Check sheet for the modelled part. Datum: model origin and axes. Units: mm. A direction names the side the tool comes from. Give positions to 0.01 mm unless a question says otherwise; leave off trailing zeros. Order: outer loops, then holes, each group sorted by start corner. A loop starts at its lowest first (then second) coordinate and runs counter-clockwise, first axis right, second up. Notation, with made-up numbers: (8.25, 25.25) -> (65.25, 25.25) arc R15 ccw to (65.25, 52.25) -> close; hole circle Ø9 at (73.25, 88.5). An arc over 180 degrees is marked (long way). One line per question, with ' | ' between items. Start each with the question number.
from build123d import *

# Parameters (mm, degrees)
SKETCH1_W                   = 50.8
SKETCH1_H                   = 50.8
STOCK_BLOCK_DEPTH           = 12.7
SKETCH2_R                   = 9.525
SLEEVE_NUT_HOLE_LARGE_DEPTH = 44.994090512
SKETCH11_W                  = 14.2875
SKETCH11_H                  = 50.8
CUT_EXTRUDE4_DEPTH          = 44.994090512
SKETCH3_W                   = 26.9875
SKETCH3_H                   = 12.7
CUT_EXTRUDE2_DEPTH          = 44.994090512
F_10_CLEARANCE_HOLE1_D      = 5.1054
SKETCH6_W                   = 3.175
SKETCH6_H                   = 37.090012852
CUT_EXTRUDE3_DEPTH          = 24.13
F_10_CLEARANCE_HOLE2_D      = 5.1054


with BuildPart() as part:
    # Sketch1 → Stock block (new, symmetric)
    with BuildSketch(Plane(origin=(0, 0, 0), x_dir=(1, 0, 0), z_dir=(0, 1, 0))):
        Rectangle(SKETCH1_W, SKETCH1_H)
    extrude(amount=STOCK_BLOCK_DEPTH, both=True)

    # Sketch2 → Sleeve Nut Hole - Large (cut, through all)
    with BuildSketch(Plane(origin=(0, 12.7, 0), x_dir=(1, 0, 0), z_dir=(0, 1, 0))):
        with Locations(Location((-7.9375, 0, 0), (0, 0, 270))):
            Circle(SKETCH2_R)
    extrude(amount=-SLEEVE_NUT_HOLE_LARGE_DEPTH, mode=Mode.SUBTRACT)

    # Sketch11 → Cut-Extrude4 (cut, through all)
    with BuildSketch(Plane(origin=(0, 12.7, 0), x_dir=(1, 0, 0), z_dir=(0, 1, 0))):
        with Locations((18.25625, 0)):
            Rectangle(SKETCH11_W, SKETCH11_H)
    extrude(amount=-CUT_EXTRUDE4_DEPTH, mode=Mode.SUBTRACT)

    # Sketch3 → Cut-Extrude2 (cut, through all)
    with BuildSketch(Plane(origin=(0, 12.7, 0), x_dir=(1, 0, 0), z_dir=(0, 1, 0))):
        with Locations((-2.38125, 19.05)):
            Rectangle(SKETCH3_W, SKETCH3_H)
        with Locations((-2.38125, -19.05)):
            Rectangle(SKETCH3_W, SKETCH3_H)
    extrude(amount=-CUT_EXTRUDE2_DEPTH, mode=Mode.SUBTRACT)

    # #10 Clearance Hole1 (through all)
    with Locations(Plane(origin=(-15.875, 0, 0), x_dir=(0, 0, -1), z_dir=(1, 0, 0))):
        with Locations((-19.05, 0), (19.05, 0)):
            Hole(F_10_CLEARANCE_HOLE1_D / 2)

    # Sketch6 → Cut-Extrude3 (cut)
    with BuildSketch(Plane(origin=(11.1125, 0, 0), x_dir=(0, 0, -1), z_dir=(1, 0, 0))):
        Rectangle(SKETCH6_W, SKETCH6_H)
    extrude(amount=-CUT_EXTRUDE3_DEPTH, mode=Mode.SUBTRACT)

    # #10 Clearance Hole2 (through all)
    with Locations(Plane.XY.offset(12.7)):
        with Locations((6.2865, 0)):
            Hole(F_10_CLEARANCE_HOLE2_D / 2)


solid = part.part
1. Go/stop test with flat-tipped pins: pin 1 (14 mm diameter, centred on y = -0.5, z = 20, fed in from +X) (3 decimals); pin 2 (2 mm diameter, centred on x = -14, y = 8, fed in from +Z); pin 3 (6.5 mm diameter, centred on x = 6.29, y = 0, fed in from -Z); pin 4 (8 mm diameter, centred on x = -12.5, y = -2, fed in from +Z). Record where each tip stops, or that it passes through.
2. Cross-section at A-A on y = 0. Give the number of separate pieces and of enclosed holes in the cut face, and give its area (3 significant figures).
3. Tool access check on faces 1 (the face through (6, 3, -1.588)), 2 (the face through (-21, 0, -25.4)), 3 (the face through (11.112, 0, -7)), 4 (the face through (-15.875, 0, 16)), 5 (the face through (-15.875, 0, -16)). Record the directions out of +Z, -Z, +X, -X, +Y, -Y that give a thin tool (end or side, any length) a straight path to the whole face; none if there is none.
4. Mould release check, pull along X, two halves, no side actions. Record for faces 6 (the face through (-17.454, 0.178, -0.396)), 7 (the face through (8.837, 0.112, -7.222)), 8 (the face through (-20.7, -1, -16.7)), 9 (the face through (-25.4, 0, 0)): +X half, -X half, draft (parallel to the pull), parting line (faces both ways), or undercut.
5. Scan lines: probe 1 along Z at (x, y) = (9.5, 2); probe 2 along Z at (x, y) = (-16, -1.5); probe 3 along X at (y, z) = (-2, 0). Record each from-to range of solid material in increasing order.
6. Cross-section at B-B on x = -19. Record the boundary of the cut face in (y, z), and give its area (3 significant figures).
7. Cross-section at C-C on z = -19.05. Record the boundary of the cut face in (x, y) (3 decimals).
Response values:
1) pin 1: stops at x = -15.875 | pin 2: stops at z = 12.7 | pin 3: stops at z = -12.7 | pin 4: stops at z = 25.4
2) separate pieces: 5 | enclosed holes: 0 | area: 643 mm²
3) face 1: +X, +Y, -Y | face 2: -Z, +X, -X, +Y, -Y | face 3: +Z, -Z, +X, +Y, -Y | face 4: +Z, +X, +Y, -Y | face 5: -Z, +X, +Y, -Y
4) face 6: undercut | face 7: undercut | face 8: draft | face 9: -X half
5) probe 1: z = -12.7 to -1.59, 1.59 to 12.7 | probe 2: z = -25.4 to -21.12, -16.98 to -5.07, 5.07 to 16.98, 21.12 to 25.4 | probe 3: x = -25.4 to -17.46
6) outline: (-12.7, -25.4) -> (12.7, -25.4) -> (12.7, 25.4) -> (-12.7, 25.4) -> close; hole circle Ø5.11 at (0, -19.05); hole circle Ø5.11 at (0, 19.05) | area: 1,250 mm²
7) outline: (-25.4, -12.7) -> (-15.875, -12.7) -> (-15.875, -2.553) -> (-25.4, -2.553) -> close; (-25.4, 2.553) -> (-15.875, 2.553) -> (-15.875, 12.7) -> (-25.4, 12.7) -> close
